Autodesk Inventor part; units mm, degrees
ref_plane "YZ Plane" through (0, 0, 0) normal (1, 0, 0) x (0, 1, 0)
ref_plane "XZ Plane" through (0, 0, 0) normal (0, 1, 0) x (-1, 0, 0)
ref_plane "XY Plane" through (0, 0, 0) normal (0, 0, 1) x (1, 0, 0)
sketch "Sketch1" plane through (0, 0, 0) normal (0, 1, 0) x (-1, 0, 0)
  circle A0 centre (0, 0) radius 9
  dimension "d0" = 18
extrude "Extrusion1" add sketch "Sketch1" along normal blind 70
sketch "Sketch2" plane through (0, 70, 0) normal (0, 1, 0) x (1, 0, 0)
  circle A0 centre (0, 0) radius 9
  circle A1 centre (0, 0) radius 8.99
  dimension "d3" = 0.01
extrude "Extrusion2" cut sketch "Sketch2" against normal blind 15
sketch "Sketch3" plane through (0, 0, 0) normal (0, -1, 0) x (1, 0, 0)
  circle A0 centre (0, 0) radius 9
  circle A1 centre (0, 0) radius 8.99
extrude "Extrusion3" cut sketch "Sketch3" against normal blind 10
thread "Thread1"
properties part number "Inductive Sensor 18mmx70mm"
Input: part model. Units: mm. Frame: model coordinates. Coordinates: 2 decimals unless noted, no trailing zeros. Loops run counter-clockwise (first coordinate to the right, second up) from the corner with the lowest first, then second, coordinate; pieces in that order, holes last. Notation, with made-up numbers: (74, 12) - (108, 12) arc R29 cw to (108, 41) - close; hole circle Ø5 at (26, 38). An arc over 180 degrees is marked (long way). Answer in a Markdown table with one row per item. Add a question column.
Item 1: Section query D-D on y = 31.5. Return the cut outline in (x, z), then the cut area to 3 significant figures.
Item 2: Contact query for flat-ended pins moving along their axis: P1, Ø1, axis at x = 3, y = 15, coming from the +Z side; P2, Ø1.5, axis at x = -7, y = 46.5, coming from the -Z side; P3, Ø5, axis at x = -4.5, y = 36, coming from the -Z side. Output: stop coordinate, or through.
Item 3: Section query C-C on y = 62.5. Return the cut outline in (x, z).
Item 4: Line query: line 1 along Z through (x, y) = (-0.5, 14); line 2 along Z through (x, y) = (-7.25, 37.5); line 3 along X through (y, z) = (43.5, -7.5). Output: solid intervals per line, ascending. Write a range as [from, to].
Recorded:
| question | item | result |
|---|---|---|
| 1 | outline | circle Ø18 at (0, 0) |
| 1 | area | 254 mm^2 |
| 2 | P1 | z = 8.65 |
| 2 | P2 | z = -6.48 |
| 2 | P3 | z = -8.77 |
| 3 | outline | circle Ø17.98 at (0, 0) |
| 4 | line 1 | [-8.99, 8.99] |
| 4 | line 2 | [-5.33, 5.33] |
| 4 | line 3 | [-4.97, 4.97] |
